For this review, take the finished solid that the model builds, in its own axes (mm). A direction names the side the tool comes from. Round coordinates to 2 decimals unless told otherwise and drop trailing zeros. Order: outer loops, then holes, each group sorted by start corner. A loop starts at its lowest first (then second) coordinate and runs counter-clockwise, first axis right, second up. Notation, with made-up numbers: M -33,-37 L 10,-37 A20 cw 10,-11 Z; hole C 9,57.5 d8. An arc over 180 degrees is marked long. Answer as a JSON object with one key per item and string values.
from build123d import *

# Parameters (mm, degrees)
F0_R     = 2.5
F1_DEPTH = 10
F2_W     = 20
F2_H     = 20
F2_R     = 2.5
F3_DEPTH = 10
F4_R     = 4
F5_SIZE  = 2


with BuildPart() as f1:
    # F0 (on Top) → F1 (new body)
    with BuildSketch(Plane.XY):
        Polygon((10, 10), (-30, 10), (-30, 0), (-30, -10), (10, -10), align=None)
        with BuildLine():
            ThreePointArc((-15.5, 0), (-17.5, -2), (-19.5, 0))
            ThreePointArc((-19.5, 0), (-17.5, 2), (-15.5, 0))
        make_face(mode=Mode.SUBTRACT)
        Circle(F0_R, mode=Mode.SUBTRACT)
    extrude(amount=F1_DEPTH)

    # F2 (on face) → F3 (join)
    with BuildSketch(Plane.XY.offset(10)):
        Rectangle(F2_W, F2_H)
        Circle(F2_R, mode=Mode.SUBTRACT)
    extrude(amount=F3_DEPTH)

    # F4
    f4_edges = [f1.edges().sort_by_distance(p)[0] for p in [
        (-30, 0, 10),
        (-20, 10, 10),
        (-20, -10, 10),
        (-10, 0, 20),
        (0, 10, 20),
        (10, 0, 20),
        (0, -10, 20),
        (-10, -10, 15),
        (-10, 10, 15),
        (10, 10, 10),
        (10, -10, 10),
        (-30, 10, 5),
        (-30, -10, 5),
    ]]
    fillet(f4_edges, radius=F4_R)

    # F5
    f5_edges = [f1.edges().sort_by_distance(p)[0] for p in [
        (-19.5, 0, 10),
    ]]
    chamfer(f5_edges, length=F5_SIZE)


solid = f1.part
1) Add section C-C on y = 5.5. State the section outline as (x, z) points.
Geometry check:
{"outline": "M -30,0 L 10,0 L 10,16 A4 ccw 6,20 L -6,20 A4 ccw -10,16 L -10,10 L -26,10 A4 ccw -30,6 Z"}
2) Add section D-D on x = -17.5. State the section outline as (y, z) points, and give its area (3 significant figures).
Geometry check:
{"outline": "M -10,0 L -2,0 L -2,8 L -4,10 L -6,10 A4 ccw -10,6 Z; M 2,0 L 10,0 L 10,6 A4 ccw 6,10 L 4,10 L 2,8 Z", "area": "149 mm²"}
3) Add section B-B on x = 0. State the section outline as (y, z) points, and give its area (3 significant figures).
Geometry check:
{"outline": "M -10,0 L -2.5,0 L -2.5,20 L -6,20 A4 ccw -10,16 Z; M 2.5,0 L 10,0 L 10,16 A4 ccw 6,20 L 2.5,20 Z", "area": "293 mm²"}
4) Mouldability with a two-part tool opening along X and no side actions: class faces 1 (the cylindrical face through (8.859, -8.797, 8.112)), 2 (the cylindrical face through (-18.082, -8.797, 8.859)), 3 (the cylindrical face through (-0.54, -2.44, 9.86)), 4 (the flat face through (-30, 0, 3)) as +X half, -X half, draft (parallel to the pull), parting line (faces both ways), or undercut.
Geometry check:
{"face 1": "+X half", "face 2": "draft", "face 3": "undercut", "face 4": "-X half"}
5) Add section A-A on y = 0. State the section outline as (x, z) points.
Geometry check:
{"outline": "M -30,0 L -19.5,0 L -19.5,8 L -21.5,10 L -26,10 A4 ccw -30,6 Z; M -15.5,0 L -2.5,0 L -2.5,20 L -6,20 A4 ccw -10,16 L -10,10 L -13.5,10 L -15.5,8 Z; M 2.5,0 L 10,0 L 10,16 A4 ccw 6,20 L 2.5,20 Z"}
6) For L1, parallel to Y at x = 1, z = 18; L2, parallel to X at y = 1.75, z = 10.5; L3, parallel to Z at x = -14, y = 4.5, list the stretches that pass through material, from the lowest coordinate up.
Geometry check:
{"L1": "y = -9.46 to -2.29, 2.29 to 9.46", "L2": "x = -10 to -1.79, 1.79 to 10", "L3": "z = 0 to 10"}
7) Machinability: for faces 5 (the cylindrical face through (-18.362, 8.797, 8.859)), 6 (the flat face through (-10, 0, 13)), 7 (the flat face through (-7, -10, 4)), which of the approach directions +Z, -Z, +X, -X, +Y, -Y give a long, thin tool a straight path to every point of the face, cutting with its end or side? Answer none if there is none.
Geometry check:
{"face 5": "+Z, -X, +Y", "face 6": "+Z, -X, +Y, -Y", "face 7": "+Z, -Z, +X, -X, -Y"}
8) Insertion check: P1, Ø3, axis at y = 0, z = 14, coming from the -X side; P2, Ø2, axis at x = -7.5, z = 10.5, coming from the +Y side; P3, Ø6, axis at x = -18, y = 0.5, coming from the +Z side. Each pin has a flat end and moves straight along its axis. Give the tip position at first contact, or say it passes through.
Geometry check:
{"P1": "stops at x = -10", "P2": "stops at y = 9.97", "P3": "stops at z = 9.71"}
